```python
from build123d import *

# Parameters (mm, degrees)
F4_R     = 2.152954
F5_DEPTH = 50.8


with BuildPart() as f1:
    # F0 (on Right) → F1 (revolve)
    with BuildSketch(Plane.YZ):
        Polygon((0, -174.897112), (0, -185.057112), (53.975, -185.057112), (53.975, -178.707112), (33.856217, -178.707112), (33.856217, -174.897112), align=None)
        Polygon((0, -165.372112), (0, -174.897112), (33.856217, -174.897112), (44.45, -165.372112), align=None)
        Polygon((44.45, -165.372112), (33.856217, -174.897112), (53.975, -174.897112), (53.975, 53.846701), (34.925, 112.763417), (34.925, 150.090903), (25.4, 150.090903), (25.4, 111.261793), (44.45, 52.345077), align=None)
    revolve(axis=Axis((0, 0, 8.948858), (0, 0, 1)))

    # F2 (on Right) → F3 (revolve)
    with BuildSketch(Plane.YZ):
        Polygon((71.640717, -70.134891), (24.463108, -105.071298), (26.635614, -108.005017), (30.627662, -105.071298), (71.058815, -75.13084), (73.798926, -73.049305), align=None)
    revolve(axis=Axis((0, 52.4091, -92.892285), (0, -0.803638, -0.595118)))

    # F4 (on face) → F5 (cut)
    with BuildSketch(Plane(origin=(0, 12.725377, 9.423516), x_dir=(-1, 0, 0), z_dir=(0, 0.803638, 0.595118))):
        with Locations((0, -105.841401)):
            Circle(F4_R)
    extrude(amount=-F5_DEPTH, mode=Mode.SUBTRACT)


solid = f1.part
```
Source: CAD feature listing. Evaluate the final solid. Frame: model axes, mm. A direction names the side the tool comes from. Coordinates: 2 decimals unless noted, no trailing zeros. Loops run counter-clockwise (first coordinate to the right, second up) from the corner with the lowest first, then second, coordinate; pieces in that order, holes last. Notation, with made-up numbers: M 62.25,59 L 83.25,59 A9 cw 83.25,70 Z; hole C -1.5,17 d7. An arc over 180 degrees is marked long. Use a Markdown table: item, result. Add a question column.
Q1. Section query B-B, the plane z = -61.5. Return loops of the section in (x, y) (3 decimals), and give its area (3 significant figures).
Q2. Section query A-A, the plane y = 0. Return loops of the section in (x, z) (3 decimals).
Q3. Access query for faces 4 (the flat face through (26, 2, 150.091)), 5 (the cylindrical face through (24.796, -5.506, 130.405)), 6 (the flat face through (35, 1, -174.897)). Directions: +Z, -Z, +X, -X, +Y, -Y. A direction counts if a zero-diameter tool reaches every point of the face in a straight line with its end or side. Return the directions, or none.
Q4. First-contact query: pin 1 (8 mm diameter, centred on y = -33, z = -115, fed in from -X); pin 2 (3 mm diameter, centred on y = 11.5, z = 30, fed in from +X); pin 3 (8 mm diameter, centred on y = 21, z = -103.5, fed in from -X). Flat tips, straight axial feed; report the tip coordinate or a pass-through.
Q5. Draft query along Y for faces 1 (the cylindrical face through (1.216, 36.244, -101.214)), 2 (the cylindrical face through (-36.48, -39.78, -181.84)), 3 (the flat face through (-1, 1, -185.057)). Return one class per face: pulls with the +Y half, pulls with the -Y half, needs draft (parallel to the pull), parting line crosses it, or undercut.
Q6. Material intervals for L1, parallel to Y at x = 0, z = 142 (3 decimals); L2, parallel to X at y = 0.5, z = -36.5, sorted ascending.
Result:
| question | item | result |
|---|---|---|
| 1 | outline | C 0,0 d107.95; hole C 0,0 d88.9 |
| 1 | area | 2,950 mm2 |
| 2 | outline | M -53.975,-185.057 L 53.975,-185.057 L 53.975,-178.707 L 33.856,-178.707 L 33.856,-174.897 L 53.975,-174.897 L 53.975,53.847 L 34.925,112.763 L 34.925,150.091 L 25.4,150.091 L 25.4,111.262 L 44.45,52.345 L 44.45,-165.372 L -44.45,-165.372 L -44.45,52.345 L -25.4,111.262 L -25.4,150.091 L -34.925,150.091 L -34.925,112.763 L -53.975,53.847 L -53.975,-174.897 L -33.856,-174.897 L -33.856,-178.707 L -53.975,-178.707 Z |
| 3 | face 4 | +Z, +X, -X, +Y, -Y |
| 3 | face 5 | +Z |
| 3 | face 6 | none |
| 4 | pin 1 | stops at x = -45.52 |
| 4 | pin 2 | stops at x = 53.04 |
| 4 | pin 3 | stops at x = -51.23 |
| 5 | face 1 | undercut |
| 5 | face 2 | parting line crosses it |
| 5 | face 3 | needs draft |
| 6 | L1 | y = -34.925 to -25.4, 25.4 to 34.925 |
| 6 | L2 | x = -53.97 to -44.45, 44.45 to 53.97 |
